```python
from build123d import *

# Parameters (mm, degrees)
EXTRUDE_1_DEPTH     = 4.4
SKETCH_1_4_W        = 0.4
SKETCH_1_4_H        = 0.4
EXTRUDE_2_DEPTH     = 4.8
SKETCH_2_R          = 1.1
EXTRUDE_3_DEPTH     = 1.6
CUT_EXTRUDE_START   = 1.6
SKETCH_2_5_W        = 0.5
SKETCH_2_5_H        = 2.2
CUT_EXTRUDE_2_DEPTH = 0.6
SKETCH_3_R          = 0.25
EXTRUDE_4_DEPTH     = 6


with BuildPart() as part:
    # 草图1 → 凸台-拉伸1 (new body)
    with BuildSketch(Plane(origin=(0, 0, 0), x_dir=(0, 0, -1), z_dir=(1, 0, 0))):
        Polygon((-4.75, 4.4), (-4.75, -4.8), (-4.35, -4.8), (4.35, -4.8), (4.75, -4.8), (4.75, 4.4), (4.35, 4.4), (4.35, 4.8), (-4.35, 4.8), (-4.35, 4.4), align=None)
    extrude(amount=EXTRUDE_1_DEPTH)

    # 草图1<4> → 凸台-拉伸2 (add)
    with BuildSketch(Plane(origin=(0, 0, 0), x_dir=(0, 0, -1), z_dir=(1, 0, 0))):
        with Locations((4.55, 4.6)):
            Rectangle(SKETCH_1_4_W, SKETCH_1_4_H)
        with Locations((4.55, -5)):
            Rectangle(SKETCH_1_4_W, SKETCH_1_4_H)
        with Locations((-4.55, 4.6)):
            Rectangle(SKETCH_1_4_W, SKETCH_1_4_H)
        with Locations((-4.55, -5)):
            Rectangle(SKETCH_1_4_W, SKETCH_1_4_H)
    extrude(amount=EXTRUDE_2_DEPTH)

    # 草图2 → 凸台-拉伸3 (add)
    with BuildSketch(Plane(origin=(0, 4.8, 0), x_dir=(1, 0, 0), z_dir=(0, 1, 0))):
        with Locations(Location((1.4, -3.65, 0), (0, 0, 270))):
            Circle(SKETCH_2_R)
    extrude(amount=EXTRUDE_3_DEPTH)

    # 草图2<5> → 切除-拉伸2 (cut)
    with BuildSketch(Plane(origin=(0, 4.8, 0), x_dir=(1, 0, 0), z_dir=(0, 1, 0)).offset(CUT_EXTRUDE_START)):
        with Locations((1.4, -3.65)):
            Rectangle(SKETCH_2_5_W, SKETCH_2_5_H)
    extrude(amount=-CUT_EXTRUDE_2_DEPTH, mode=Mode.SUBTRACT)

    # 草图3 → 凸台-拉伸4 (add)
    with BuildSketch(Plane.XZ.offset(4.8)):
        with Locations(Location((2.2, 0, 0), (0, 0, 90))):
            Circle(SKETCH_3_R)
        with Locations(Location((2.2, 2.5, 0), (0, 0, 90))):
            Circle(SKETCH_3_R)
        with Locations(Location((2.2, -2.5, 0), (0, 0, 90))):
            Circle(SKETCH_3_R)
    extrude(amount=EXTRUDE_4_DEPTH)


solid = part.part
```
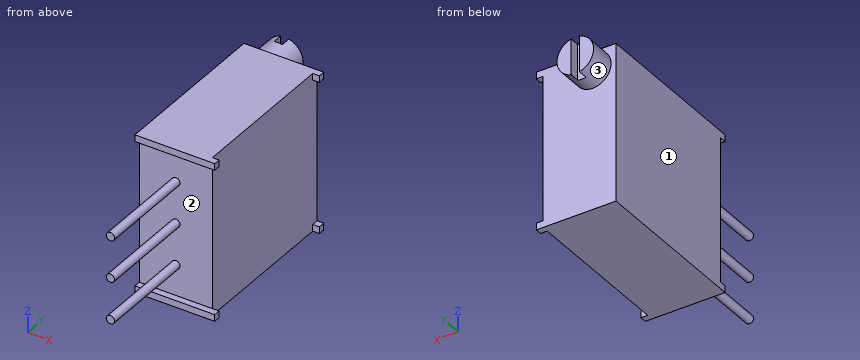
Input: part model. Units: mm. Frame: model coordinates. Face numbers are marked on the shaded views. Round coordinates to 2 decimals unless told otherwise and drop trailing zeros. Loops run counter-clockwise (first coordinate to the right, second up) from the corner with the lowest first, then second, coordinate; pieces in that order, holes last. Notation, with made-up numbers: M 9,-6.75 L 47,-6.75 A22 ccw 47,19.25 Z; hole C -2,49 d5. An arc over 180 degrees is marked long. Answer in a Markdown table with one row per item. Add a question column.
1. Ray query, probe 1 along Y at (x, z) = (4.1, 2.5); probe 2 along Y at (x, z) = (0.55, 4); probe 3 along X at (y, z) = (-3.25, 3.5). Return the intervals inside material, ascending.
2. Section B-B (z = 3.65). Output: boundary loops of the cut face in (x, y).
3. Mould query, pull axis Z, two halves, no side actions, for the marked faces 1, 2 and 3. Classes: released by +Z, released by -Z, zero draft, split by the parting line, or undercut.
4. Section A-A (y = -5.5). Output: boundary loops of the cut face in (x, z).
5. Contact query for flat-ended pins moving along their axis: pin 1 (5 mm diameter, centred on y = 2.5, z = 2.5, fed in from -X); pin 2 (3 mm diameter, centred on y = 1.5, z = 2, fed in from +X); pin 3 (1.3 mm diameter, centred on x = 2, z = 1, fed in from -Y); pin 4 (0.7 mm diameter, centred on y = 6, z = 3.5, fed in from -X). Output: stop coordinate, or through.
6. Section C-C (y = 3). Output: boundary loops of the cut face in (x, z).
7. Section D-D (x = 0.8). Output: boundary loops of the cut face in (y, z).
Values follow:
| question | item | result |
|---|---|---|
| 1 | probe 1 | -4.8 to 4.8 |
| 1 | probe 2 | -4.8 to 6.4 |
| 1 | probe 3 | 0 to 4.4 |
| 2 | outline | M 0,-4.8 L 4.4,-4.8 L 4.4,4.8 L 2.5,4.8 L 2.5,6.4 L 1.65,6.4 L 1.65,5.8 L 1.15,5.8 L 1.15,6.4 L 0.3,6.4 L 0.3,4.8 L 0,4.8 Z |
| 3 | face 1 | zero draft |
| 3 | face 2 | undercut |
| 3 | face 3 | split by the parting line |
| 4 | outline | C 2.2,-2.5 d0.5; C 2.2,0 d0.5; C 2.2,2.5 d0.5 |
| 5 | pin 1 | x = 0 |
| 5 | pin 2 | x = 4.4 |
| 5 | pin 3 | y = -4.8 |
| 5 | pin 4 | x = 0.3 |
| 6 | outline | M 0,-4.75 L 4.4,-4.75 L 4.4,4.75 L 0,4.75 Z |
| 7 | outline | M -5.2,-4.75 L 4.8,-4.75 L 4.8,2.73 L 6.4,2.73 L 6.4,4.57 L 4.8,4.57 L 4.8,4.75 L -5.2,4.75 L -5.2,4.35 L -4.8,4.35 L -4.8,-4.35 L -5.2,-4.35 Z |
